Verification items for this drawing (mm, ordinates from the low corner). A direction names the side the tool comes from. Give positions to 0.01 mm unless a question says otherwise; leave off trailing zeros. Write each loop counter-clockwise with the first axis right and the second up, starting at its lowest first coordinate (ties: lowest second). Pieces come first, ordered by that corner, then holes. Notation, with made-up numbers: (-14.5, 18) -> (-0.5, 18) arc R13 ccw to (-0.5, 24) -> close; hole circle Ø3 at (-30, 70). An arc over 180 degrees is marked (long way). Answer as a JSON object with one key per item and string values.
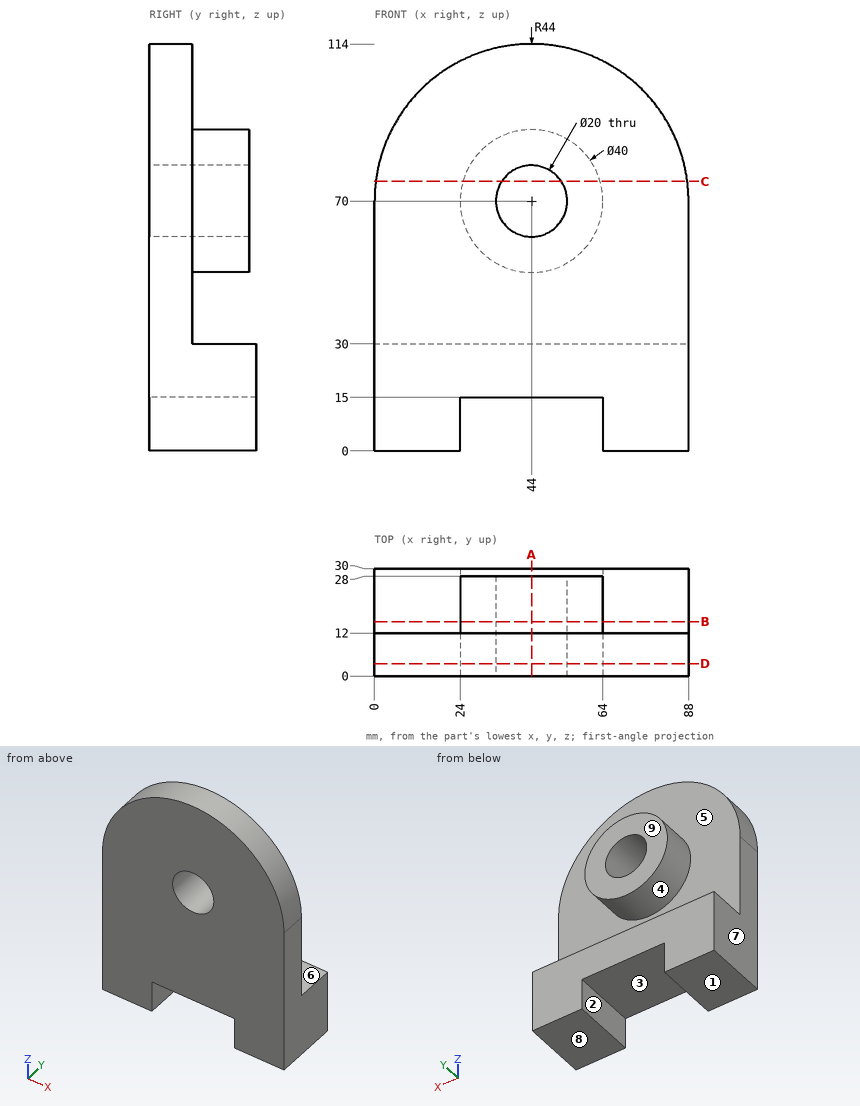
1. Go/stop test with flat-tipped pins: P1, Ø14.5, axis at x = 44.5, y = 21, coming from the +Z side; P2, Ø1.5, axis at x = 38, y = 12, coming from the +Z side; P3, Ø5, axis at x = 20, y = 20, coming from the +Z side; P4, Ø18, axis at x = 44, z = 70, coming from the -Y side. Record where each tip stops, or that it passes through.
Determined:
{"P1": "z = 90", "P2": "z = 113.69", "P3": "z = 30", "P4": "through"}
2. Scan lines: L1, parallel to Z at x = 44, y = 14; L2, parallel to Z at x = 44, y = 6; L3, parallel to Z at x = 35, y = 19. Record each from-to range of solid material in increasing order. Write a range as [from, to].
Determined:
{"L1": "[15, 30], [50, 60], [80, 90]", "L2": "[15, 60], [80, 114]", "L3": "[15, 30], [52.14, 65.64], [74.36, 87.86]"}
3. Sectioned sample at B-B, the plane y = 15.25. Enter the section's corners in (x, z).
Determined:
{"outline": "(0, 0) -> (24, 0) -> (24, 15) -> (64, 15) -> (64, 0) -> (88, 0) -> (88, 30) -> (0, 30) -> close; circle Ø40 at (44, 70); hole circle Ø20 at (44, 70)"}
4. Access from +Z, -Z, +X, -X, +Y, -Y to the whole of each face (thin tool, end or side, straight path). Record for the marked faces 5, 6, 7, 8 and 9.
Determined:
{"face 5": "+Y", "face 6": "+X, -X, +Y", "face 7": "+Z, -Z, -X, +Y, -Y", "face 8": "-Z, +X, -X, +Y, -Y", "face 9": "+Z, +X, -X, +Y"}
5. Sectioned sample at C-C, the plane z = 75.5. Enter the section's corners in (x, y).
Determined:
{"outline": "(0.35, 0) -> (35.65, 0) -> (35.65, 28) -> (24.77, 28) -> (24.77, 12) -> (0.35, 12) -> close; (52.35, 0) -> (87.65, 0) -> (87.65, 12) -> (63.23, 12) -> (63.23, 28) -> (52.35, 28) -> close"}
6. Mould release check, pull along X, two halves, no side actions. Record for the marked faces 1, 2, 3 and 4: released by +X, released by -X, zero draft, split by the parting line, or undercut.
Determined:
{"face 1": "zero draft", "face 2": "undercut", "face 3": "undercut", "face 4": "split by the parting line"}
7. Sectioned sample at D-D, the plane y = 3.5. Enter the section's corners in (x, z).
Determined:
{"outline": "(0, 0) -> (24, 0) -> (24, 15) -> (64, 15) -> (64, 0) -> (88, 0) -> (88, 70) arc R44 ccw to (0, 70) -> close; hole circle Ø20 at (44, 70)"}
8. Sectioned sample at A-A, the plane x = 44. Enter the section's corners in (y, z), plus the area to 3 significant figures.
Determined:
{"outline": "(0, 15) -> (30, 15) -> (30, 30) -> (12, 30) -> (12, 50) -> (28, 50) -> (28, 60) -> (0, 60) -> close; (0, 80) -> (28, 80) -> (28, 90) -> (12, 90) -> (12, 114) -> (0, 114) -> close", "area": "1,540 mm^2"}
